Input: part model. Units: mm. Frame: model coordinates. Face numbers are marked on the shaded views. A direction names the side the tool comes from. Give positions to 0.01 mm unless a question says otherwise; leave off trailing zeros. Loops run counter-clockwise (first coordinate to the right, second up) from the corner with the lowest first, then second, coordinate; pieces in that order, holes last. Notation, with made-up numbers: M 30.25,87.25 L 37.25,87.25 A9 ccw 37.25,102.25 Z; hole C 82.5,20 d9. An arc over 180 degrees is marked long. Answer as a JSON object with one key per item and string values. Group by question number.
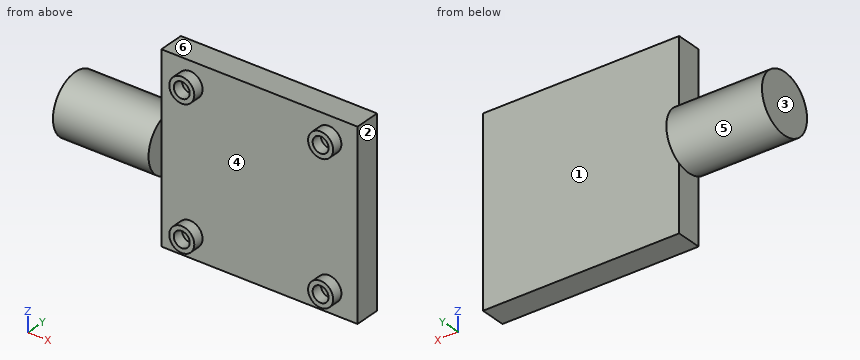
```python
from build123d import *

# Parameters (mm, degrees)
SKETCH1_W           = 43.1
SKETCH1_H           = 40.3
BOSS_EXTRUDE1_DEPTH = 5.62
SKETCH2_R           = 2.75
SKETCH2_R_2         = 1.75
BOSS_EXTRUDE2_DEPTH = 8
SKETCH3_R           = 6.5
BOSS_EXTRUDE3_DEPTH = 21


with BuildPart() as part:
    # Sketch1 → Boss-Extrude1 (new body)
    with BuildSketch(Plane(origin=(0, 0, 0), x_dir=(1, 0, 0), z_dir=(0, 1, 0))):
        Rectangle(SKETCH1_W, SKETCH1_H)
    extrude(amount=BOSS_EXTRUDE1_DEPTH)

    # Sketch2 → Boss-Extrude2 (add)
    with BuildSketch(Plane(origin=(0, 5.62, 0), x_dir=(1, 0, 0), z_dir=(0, 1, 0))):
        with Locations((-15.25, 15.25)):
            Circle(SKETCH2_R)
        with Locations((-15.25, 15.25)):
            Circle(SKETCH2_R_2, mode=Mode.SUBTRACT)
        with Locations((15.25, 15.25)):
            Circle(SKETCH2_R)
        with Locations((15.25, 15.25)):
            Circle(SKETCH2_R_2, mode=Mode.SUBTRACT)
        with Locations((15.25, -15.25)):
            Circle(SKETCH2_R)
        with Locations((15.25, -15.25)):
            Circle(SKETCH2_R_2, mode=Mode.SUBTRACT)
        with Locations((-15.25, -15.25)):
            Circle(SKETCH2_R)
        with Locations((-15.25, -15.25)):
            Circle(SKETCH2_R_2, mode=Mode.SUBTRACT)
    extrude(amount=-BOSS_EXTRUDE2_DEPTH)

    # Sketch3 → Boss-Extrude3 (add)
    with BuildSketch(Plane.ZY.offset(21.55)):
        with Locations((0, 2.81)):
            Circle(SKETCH3_R)
    extrude(amount=BOSS_EXTRUDE3_DEPTH)


solid = part.part
```
1. First-contact query: P1, Ø2, axis at x = 15.25, z = -15.25, coming from the +Y side; P2, Ø4.5, axis at x = -14, z = 14.5, coming from the -Y side; P3, Ø6, axis at y = 2.5, z = 14.5, coming from the -X side. Flat tips, straight axial feed; report the tip coordinate or a pass-through.
2. Material intervals for L1, parallel to X at y = -1.2, z = 15.25; L2, parallel to Y at x = 1.5, z = -7.5, sorted ascending.
3. Section B-B (z = 15.25). Output: boundary loops of the cut face in (x, y).
4. Section A-A (y = -1.5). Count the separate pieces of the cut face and the enclosed holes in it, then the cut area to 3 significant figures.
5. Section D-D (y = 2.81). Output: boundary loops of the cut face in (x, z).
6. Mould query, pull axis Z, two halves, no side actions, for the marked faces 3, 4, 5 and 6. Classes: pulls with the +Z half, pulls with the -Z half, needs draft (parallel to the pull), parting line crosses it, or undercut.
7. Reachability of the marked faces 1 and 2 from +Z, -Z, +X, -X, +Y, -Y: full face, straight path, thin tool, end or side. Return the list, or none.
8. Section C-C (x = 15.25). Output: boundary loops of the cut face in (y, z).
Geometry results:
{
 "1": {"P1": "y = 5.62", "P2": "y = -2.38", "P3": "x = -21.55"},
 "2": {"L1": "-18 to -17, -13.5 to -12.5, 12.5 to 13.5, 17 to 18", "L2": "0 to 5.62"},
 "3": {"outline": "M -21.55,0 L -18,0 L -18,-2.38 L -17,-2.38 L -17,0 L -13.5,0 L -13.5,-2.38 L -12.5,-2.38 L -12.5,0 L 12.5,0 L 12.5,-2.38 L 13.5,-2.38 L 13.5,0 L 17,0 L 17,-2.38 L 18,-2.38 L 18,0 L 21.55,0 L 21.55,5.62 L -21.55,5.62 Z"},
 "4": {"separate pieces": "5", "enclosed holes": "4", "area": "261 mm2"},
 "5": {"outline": "M -42.55,-6.5 L -21.55,-6.5 L -21.55,-20.15 L 21.55,-20.15 L 21.55,20.15 L -21.55,20.15 L -21.55,6.5 L -42.55,6.5 Z"},
 "6": {"face 3": "needs draft", "face 4": "undercut", "face 5": "parting line crosses it", "face 6": "pulls with the +Z half"},
 "7": {"face 1": "+Z, -Z, +X, +Y", "face 2": "+Z, -Z, +X, +Y, -Y"},
 "8": {"outline": "M -2.38,-18 L 0,-18 L 0,-20.15 L 5.62,-20.15 L 5.62,20.15 L 0,20.15 L 0,18 L -2.38,18 L -2.38,17 L 0,17 L 0,13.5 L -2.38,13.5 L -2.38,12.5 L 0,12.5 L 0,-12.5 L -2.38,-12.5 L -2.38,-13.5 L 0,-13.5 L 0,-17 L -2.38,-17 Z"}
}
